Geometry: final body of the model. Coordinates: model frame, mm. Face numbers are marked on the shaded views. A direction names the side the tool comes from. Give positions to 0.01 mm unless a question says otherwise; leave off trailing zeros. Write each loop counter-clockwise with the first axis right and the second up, starting at its lowest first coordinate (ties: lowest second). Pieces come first, ordered by that corner, then holes.
from build123d import *

# Parameters (mm, degrees)
BOSS_EXTRUDE2_DEPTH = 40
SKETCH3_R           = 4.125
CUT_EXTRUDE1_DEPTH  = 38
CHAMFER1_SIZE       = 0.5
CHAMFER1_SIZE2      = 0.866025404


with BuildPart() as part:
    # Sketch2 → Boss-Extrude2 (new body)
    with BuildSketch(Plane(origin=(0, 0, 0), x_dir=(1, 0, 0), z_dir=(0, 1, 0))):
        Polygon((-31.312103746, 37), (-31.312103746, 0), (48.687896254, 0), (48.687896254, 37), (28.787896254, 37), (28.787896254, 17.4), (-11.412103746, 17.4), (-11.412103746, 37), align=None)
    extrude(amount=BOSS_EXTRUDE2_DEPTH)

    # Sketch3 → Cut-Extrude1 (cut, through all)
    with BuildSketch(Plane.XY):
        with Locations((-3.812103746, 31.5)):
            Circle(SKETCH3_R)
        with Locations((21.187896254, 31.5)):
            Circle(SKETCH3_R)
        with Locations((21.187896254, 8.5)):
            Circle(SKETCH3_R)
        with Locations((-3.812103746, 8.5)):
            Circle(SKETCH3_R)
        with Locations((-21.312103746, 31.5)):
            Circle(SKETCH3_R)
        with Locations((38.687896254, 31.5)):
            Circle(SKETCH3_R)
        with Locations((38.687896254, 8.5)):
            Circle(SKETCH3_R)
        with Locations((-21.312103746, 8.5)):
            Circle(SKETCH3_R)
        with Locations((8.687896254, 20)):
            Circle(SKETCH3_R)
    extrude(amount=-CUT_EXTRUDE1_DEPTH, mode=Mode.SUBTRACT)

    # Chamfer1
    chamfer1_edges = [part.edges().sort_by_distance(p)[0] for p in [
        (-7.937103746, 31.5, 0),
        (4.562896254, 20, 0),
        (-25.437103746, 8.5, 0),
        (34.562896254, 8.5, 0),
        (34.562896254, 31.5, 0),
        (-25.437103746, 31.5, 0),
        (-7.937103746, 8.5, 0),
        (17.062896254, 8.5, 0),
        (17.062896254, 31.5, 0),
    ]]
    chamfer1_side = [part.faces().sort_by_distance(p)[0] for p in [
        (-30.417676555, 20, 0),
    ]]
    chamfer(chamfer1_edges, length=CHAMFER1_SIZE, length2=CHAMFER1_SIZE2, reference=chamfer1_side[0])


solid = part.part
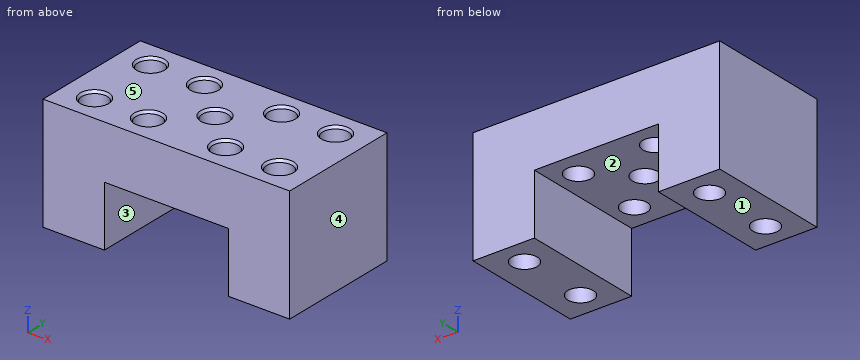
Q1. Ray query, line 1 along Y through (x, z) = (-21, -24); line 2 along X through (y, z) = (13, -26); line 3 along X through (y, z) = (34, -8.5). Return the intervals inside material, ascending.
Filled sheet:
line 1: y = 0 to 4.39, 12.61 to 27.39, 35.61 to 40
line 2: x = -31.31 to -11.41, 28.79 to 48.69
line 3: x = -31.31 to -24.59, -18.03 to -7.09, -0.53 to 17.91, 24.47 to 35.41, 41.97 to 48.69
Q2. Pull-direction query (X, two-part tool) for the marked faces 3, 4 and 5; classes: released by +X, released by -X, zero draft, split by the parting line, or undercut.
Filled sheet:
face 3: undercut
face 4: released by +X
face 5: zero draft
Q3. Section B-B on y = 20. Output: boundary loops of the cut face in (x, z).
Filled sheet:
outline: (-31.31, -37) - (-11.41, -37) - (-11.41, -17.4) - (4.56, -17.4) - (4.56, -0.87) - (4.06, 0) - (-31.31, 0) - close; (12.81, -17.4) - (28.79, -17.4) - (28.79, -37) - (48.69, -37) - (48.69, 0) - (13.31, 0) - (12.81, -0.87) - close
Q4. Access query for the marked faces 1 and 2. Directions: +Z, -Z, +X, -X, +Y, -Y. A direction counts if a zero-diameter tool reaches every point of the face in a straight line with its end or side. Return the directions, or none.
Filled sheet:
face 1: -Z, +X, -X, +Y, -Y
face 2: -Z, +Y, -Y
Q5. Section A-A on z = -21.5. Output: boundary loops of the cut face in (x, y) (3 decimals).
Filled sheet:
outline: (-31.312, 0) - (-11.412, 0) - (-11.412, 40) - (-31.312, 40) - close; (28.788, 0) - (48.688, 0) - (48.688, 40) - (28.788, 40) - close; hole circle Ø8.25 at (-21.312, 8.5); hole circle Ø8.25 at (-21.312, 31.5); hole circle Ø8.25 at (38.688, 8.5); hole circle Ø8.25 at (38.688, 31.5)
Q6. Section C-C on y = 8.5. Count the separate pieces of the cut face and the enclosed holes in it, plus the area to 3 significant figures.
Filled sheet:
separate pieces: 5
enclosed holes: 0
area: 1,270 mm2
Q7. Pin query (flat end, axial travel): P1, Ø12, axis at x = 1, y = 14, coming from the -Z side; P2, Ø7.5, axis at x = -3.81, y = 31.5, coming from the -Z side. Return the tip coordinate at first contact, or that it passes through.
Filled sheet:
P1: stops at z = -17.4
P2: passes through
